```python
from build123d import *

# Parameters (mm, degrees)
F0_W     = 150
F0_H     = 25
F0_R     = 2
F1_DEPTH = 55
F2_W     = 12
F2_H     = 5
F3_DEPTH = 150.001
F4_W     = 63.65
F4_H     = 45
F4_W_2   = 12.7
F4_H_2   = 12
F5_DEPTH = 25.001
F7_DEPTH = 86.351
F6_R     = 7.5
F8_DEPTH = 86.351
F9_R     = 4.99999
F10_SIZE = 1.5


# Not quite as in the source:
# - a fillet or chamfer is up to 0.001 mm smaller than in the source, because OpenCascade refuses the exact size


with BuildPart() as f1:
    # F0 (on Top) → F1 (new body)
    with BuildSketch(Plane.XY):
        Rectangle(F0_W, F0_H)
        with Locations((0, -7.5)):
            Circle(F0_R, mode=Mode.SUBTRACT)
        with Locations((-50, 0)):
            Circle(F0_R, mode=Mode.SUBTRACT)
        with Locations((50, 0)):
            Circle(F0_R, mode=Mode.SUBTRACT)
        with Locations((0, 7.5)):
            Circle(F0_R, mode=Mode.SUBTRACT)
    extrude(amount=F1_DEPTH)

    # F2 (on face) → F3 (cut, through all)
    with BuildSketch(Plane.YZ.offset(75)):
        with Locations((0, 52.5)):
            Rectangle(F2_W, F2_H)
    extrude(amount=-F3_DEPTH, mode=Mode.SUBTRACT)

    # F4 (on face) → F5 (cut, through all)
    with BuildSketch(Plane.XZ.offset(12.5)):
        with Locations((43.175, 22.5)):
            Rectangle(F4_W, F4_H)
        with Locations((-43.175, 22.5)):
            Rectangle(F4_W, F4_H)
        with Locations((0, 6)):
            Rectangle(F4_W_2, F4_H_2)
    extrude(amount=-F5_DEPTH, mode=Mode.SUBTRACT)

    # F6 (on face) → F7 (cut, through all)
    with BuildSketch(Plane(origin=(-11.35, 0, 0), x_dir=(0, -1, 0), z_dir=(-1, 0, 0))):
        with BuildLine():
            Line((-7.5, 0), (7.5, 0))
            ThreePointArc((7.5, 0), (0, 7.5), (-7.5, 0))
        make_face()
    extrude(amount=-F7_DEPTH, mode=Mode.SUBTRACT)

    # F6 (on face) → F8 (cut, through all)
    with BuildSketch(Plane(origin=(-11.35, 0, 0), x_dir=(0, -1, 0), z_dir=(-1, 0, 0))):
        with Locations((0, 30)):
            Circle(F6_R)
    extrude(amount=-F8_DEPTH, mode=Mode.SUBTRACT)

    # F9 (radius 5 in the source; OpenCascade refuses exactly that, so slightly less here)
    f9_edges = [f1.edges().sort_by_distance(p)[0] for p in [
        (-11.35, 7.5, 30),
        (11.35, 7.5, 30),
    ]]
    fillet(f9_edges, radius=F9_R)

    # F10
    f10_edges = [f1.edges().sort_by_distance(p)[0] for p in [
        (48, 0, 45),
        (-52, 0, 45),
    ]]
    chamfer(f10_edges, length=F10_SIZE)


solid = f1.part
```
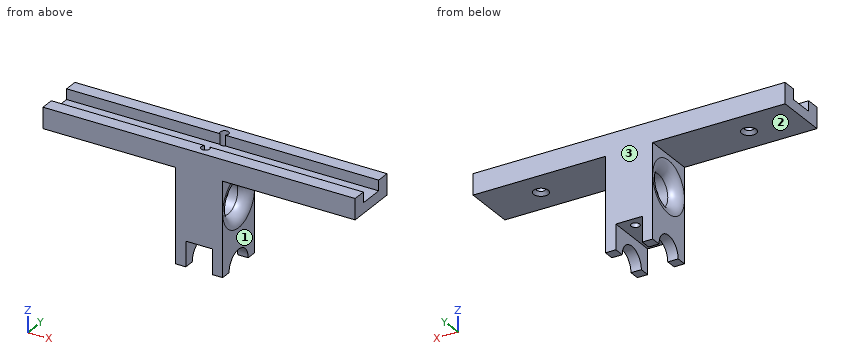
Input: part model. Units: mm. Frame: model coordinates. Face numbers are marked on the shaded views. A direction names the side the tool comes from. Give positions to 0.01 mm unless a question says otherwise; leave off trailing zeros. Loops run counter-clockwise (first coordinate to the right, second up) from the corner with the lowest first, then second, coordinate; pieces in that order, holes last. Notation, with made-up numbers: (74, 76) -> (107, 76) arc R19 cw to (107, 93) -> close; hole circle Ø1 at (-28.75, 46.25). An arc over 180 degrees is marked (long way). Use a Markdown table: item, result.
Q1. Access query for the marked faces 1, 2 and 3. Directions: +Z, -Z, +X, -X, +Y, -Y. A direction counts if a zero-diameter tool reaches every point of the face in a straight line with its end or side. Return the directions, or none.
Entries:
| item | result |
|---|---|
| face 1 | -Z, +X, +Y, -Y |
| face 2 | -Z, -X, +Y, -Y |
| face 3 | +Z, -Z, +X, -X, +Y |
Q2. First-contact query: P1, Ø13, axis at y = 5, z = 4, coming from the +X side; P2, Ø3.5, axis at x = -2, y = 1.5, coming from the +Z side; P3, Ø3.5, axis at y = 6, z = 7, coming from the -X side. Flat tips, straight axial feed; report the tip coordinate or a pass-through.
Entries:
| item | result |
|---|---|
| P1 | stops at x = 11.35 |
| P2 | stops at z = 50 |
| P3 | stops at x = -11.35 |
Q3. Section query C-C, the plane x = 65. Return the cut outline in (y, z).
Entries:
| item | result |
|---|---|
| outline | (-12.5, 45) -> (12.5, 45) -> (12.5, 55) -> (6, 55) -> (6, 50) -> (-6, 50) -> (-6, 55) -> (-12.5, 55) -> close |
Q4. Section query D-D, the plane z = 15. Return the cut outline in (x, y), plus the area to 3 significant figures.
Entries:
| item | result |
|---|---|
| outline | (-11.35, -12.5) -> (11.35, -12.5) -> (11.35, 12.5) -> (-11.35, 12.5) -> close; hole circle Ø4 at (0, -7.5); hole circle Ø4 at (0, 7.5) |
| area | 542 mm² |
Q5. Ray query, probe 1 along X at (y, z) = (0, 47.6); probe 2 along Y at (x, z) = (0, 38); probe 3 along Z at (x, y) = (1.75, 0). Return the intervals inside material, ascending. Write a range as from..to.
Entries:
| item | result |
|---|---|
| probe 1 | x = -75..-52, -48..48, 52..75 |
| probe 2 | y = -12.5..-9.5, -5.5..5.5, 9.5..12.5 |
| probe 3 | z = 12..22.5, 37.5..50 |
Q6. Section query B-B, the plane x = 50. Return the cut outline in (y, z), plus the area to 3 significant figures.
Entries:
| item | result |
|---|---|
| outline | (-12.5, 45) -> (-3.5, 45) -> (-2, 46.5) -> (-2, 50) -> (-6, 50) -> (-6, 55) -> (-12.5, 55) -> close; (2, 46.5) -> (3.5, 45) -> (12.5, 45) -> (12.5, 55) -> (6, 55) -> (6, 50) -> (2, 50) -> close |
| area | 168 mm² |
